The listing builds one solid part. Answer for the finished solid, in the listing's coordinates (mm). Face numbers are marked on the shaded views. Coordinates: 2 decimals unless noted, no trailing zeros. Order: outer loops, then holes, each group sorted by start corner. A loop starts at its lowest first (then second) coordinate and runs counter-clockwise, first axis right, second up. Notation, with made-up numbers: M -10,-15 L 30,-15 A19 ccw 30,6 Z; hole C 24.5,-3 d6. An arc over 180 degrees is marked long. One line per item, written item: value. Start each with the question number.
Q1. The part is cut by section C-C on y = -3. Give the vertices of the cut face in (x, z), then the cut area to 3 significant figures.
Q2. Each of these flat-tipped pins is pushed along its axis until it touches: pin 1 Ø3 at (y, z) = (-11, 17.5) entering from -X; pin 2 Ø4 at (y, z) = (2, 19.5) entering from -X; pin 3 Ø10 at (x, z) = (6, 17.5) entering from +Y; pin 4 Ø8 at (x, z) = (16.5, 3) entering from -Y. Where does it stop, or does it pass through?
Q3. Straight lines are drawn through the part: line 1 along X through (y, z) = (-2, 14); line 2 along X through (y, z) = (5, 23.75); line 3 along Y through (x, z) = (2.5, 20). For each, find the intervals that lie inside material, in ascending order. Write a range as [from, to].
Q4. Determine the mould class of the marked faces 1, 2 and 3 for opening direction Y: pulls with the +Y half, pulls with the -Y half, needs draft (parallel to the pull), parting line crosses it, or undercut.
Q5. The part is cut by section B-B on y = 8.5. Give the vertices of the cut face in (x, z), then the cut area to 3 significant figures.
Q6. The part is cut by section A-A on z = 15.75. Give the number of separate pieces and of enclosed holes in the cut face, then the cut area to 3 significant figures.
Q7. The part is cut by section D-D on y = 5.5. Give the vertices of the cut face in (x, z).
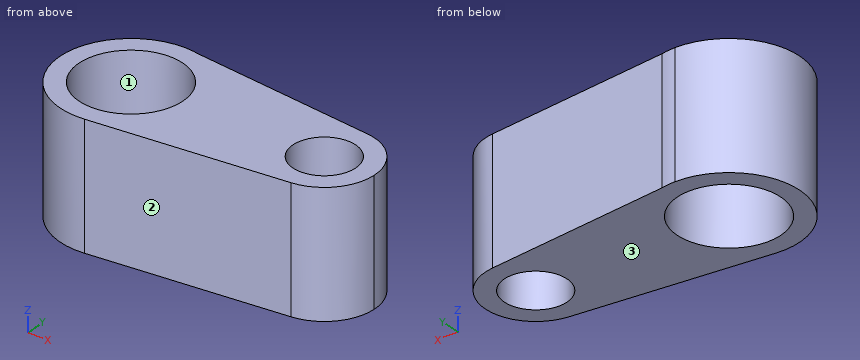
```python
from build123d import *

# Parameters (mm, degrees)
F0_R     = 10.4775
F0_R_2   = 6.35
F1_DEPTH = 25


with BuildPart() as f1:
    # F0 (on Top) → F1 (new body)
    with BuildSketch(Plane.XY):
        with BuildLine():
            Line((2.903655, 13.989333), (0, 14.2875))
            ThreePointArc((0, 14.2875), (-14.268105, -0.744198), (1.486376, -14.209973))
            ThreePointArc((1.486376, -14.209973), (10.615301, -9.562846), (14.2875, 0))
            ThreePointArc((14.2875, 0), (11.081936, 9.017946), (2.903655, 13.989333))
        make_face()
        Circle(F0_R, mode=Mode.SUBTRACT)
        with BuildLine():
            ThreePointArc((2.903655, 13.989333), (1.459462, 14.212763), (0, 14.2875))
            Line((0, 14.2875), (2.903655, 13.989333))
        make_face()
        with BuildLine():
            ThreePointArc((14.2875, 0), (10.615301, -9.562846), (1.486376, -14.209973))
            Line((1.486376, -14.209973), (40.731778, -10.10487))
            ThreePointArc((40.731778, -10.10487), (29.514805, -0.009621), (40.712639, 10.106854))
            Line((40.712639, 10.106854), (2.903655, 13.989333))
            ThreePointArc((2.903655, 13.989333), (11.081936, 9.017946), (14.2875, 0))
        make_face()
        with BuildLine():
            ThreePointArc((40.712639, 10.106854), (29.514805, -0.009621), (40.731778, -10.10487))
            ThreePointArc((40.731778, -10.10487), (47.223459, -6.800246), (49.8348, 0))
            ThreePointArc((49.8348, 0), (47.217016, 6.807391), (40.712639, 10.106854))
        make_face()
        with Locations((39.6748, 0)):
            Circle(F0_R_2, mode=Mode.SUBTRACT)
    extrude(amount=F1_DEPTH)


solid = f1.part
```
Output:
1. outline: M -13.97,0 L -10.04,0 L -10.04,25 L -13.97,25 Z; M 10.04,0 L 34.08,0 L 34.08,25 L 10.04,25 Z; M 45.27,0 L 49.38,0 L 49.38,25 L 45.27,25 Z
1. area: 802 mm^2
2. pin 1: stops at x = -10.67
2. pin 2: stops at x = -14.29
2. pin 3: stops at y = 14.25
2. pin 4: stops at y = -13.06
3. line 1: x = [-14.15, -10.28], [10.28, 33.65], [45.7, 49.64]
3. line 2: x = [-13.38, -9.21], [9.21, 35.76], [43.59, 48.52]
3. line 3: y = [-14.1, -10.17], [10.17, 14.07]
4. face 1: undercut
4. face 2: pulls with the -Y half
4. face 3: needs draft
5. outline: M -11.48,0 L -6.13,0 L -6.13,25 L -11.48,25 Z; M 6.13,0 L 45.24,0 L 45.24,25 L 6.13,25 Z
5. area: 1,110 mm^2
6. separate pieces: 1
6. enclosed holes: 2
6. area: 985 mm^2
7. outline: M -13.19,0 L -8.92,0 L -8.92,25 L -13.19,25 Z; M 8.92,0 L 36.5,0 L 36.5,25 L 8.92,25 Z; M 42.85,0 L 48.22,0 L 48.22,25 L 42.85,25 Z
